```python
from build123d import *

# Parameters (mm, degrees)
SKETCH_1_W                  = 220
SKETCH_1_H                  = 220
EXTRUDE_2_DEPTH             = 220
SKETCH_3_R                  = 78
CUT_EXTRUDE_1_DEPTH         = 240
SHELL_2_T                   = 3
SKETCH_5_W                  = 207.122367347
SKETCH_5_H                  = 195.284428571
CUT_EXTRUDE_3_DEPTH         = 180
SKETCH_12_W                 = 226
SKETCH_12_H                 = 223
CUT_EXTRUDE_6_DEPTH         = 3
SKETCH_13_W                 = 226
SKETCH_13_H                 = 223
CUT_EXTRUDE_7_DEPTH         = 3
EXTRUDE_6_REACH             = 272.682
SKETCH_16_W                 = 40
SKETCH_16_H                 = 5
EXTRUDE_6_DIRECTION_2_REACH = 272.682


with BuildPart() as part:
    # 草图1 → 凸台-拉伸2 (new body)
    with BuildSketch(Plane(origin=(0, 0, 0), x_dir=(1, 0, 0), z_dir=(0, 1, 0))):
        Rectangle(SKETCH_1_W, SKETCH_1_H)
    extrude(amount=EXTRUDE_2_DEPTH)

    # 草图3 → 切除-拉伸1 (cut)
    with BuildSketch(Plane(origin=(0, 0, 0), x_dir=(1, 0, 0), z_dir=(0, 1, 0))):
        with Locations(Location((0, 0, 0), (0, 0, 270))):
            Circle(SKETCH_3_R)
    extrude(amount=CUT_EXTRUDE_1_DEPTH, mode=Mode.SUBTRACT)

    # 抽壳2
    shell_2_openings = [part.faces().sort_by_distance(p)[0] for p in [
        (0, 220, -106.888730163),
    ]]
    offset(amount=SHELL_2_T, openings=shell_2_openings, kind=Kind.INTERSECTION)

    # 草图5 → 切除-拉伸3 (cut)
    with BuildSketch(Plane.ZY.offset(-78)):
        with Locations((-1.991561224, 122.357785714)):
            Rectangle(SKETCH_5_W, SKETCH_5_H)
    extrude(amount=CUT_EXTRUDE_3_DEPTH, mode=Mode.SUBTRACT)

    # 草图12 → 切除-拉伸6 (cut)
    with BuildSketch(Plane(origin=(113, 0, 0), x_dir=(0, 0, -1), z_dir=(1, 0, 0))):
        with Locations((0, 108.5)):
            Rectangle(SKETCH_12_W, SKETCH_12_H)
    extrude(amount=-CUT_EXTRUDE_6_DEPTH, mode=Mode.SUBTRACT)

    # 草图13 → 切除-拉伸7 (cut)
    with BuildSketch(Plane.ZY.offset(113)):
        with Locations((0, 108.5)):
            Rectangle(SKETCH_13_W, SKETCH_13_H)
    extrude(amount=-CUT_EXTRUDE_7_DEPTH, mode=Mode.SUBTRACT)

    # 凸台-拉伸6: up to this face of the body (flat: up to its plane)
    extrude_6_end = Plane(part.part.faces().sort_by_distance((0, 110, -110))[0])
    # 草图16 → 凸台-拉伸6 (add, up to the picked face)
    with BuildSketch(Plane.XY, mode=Mode.PRIVATE) as extrude_6_sk1:
        with Locations((-35, 164.5)):
            Rectangle(SKETCH_16_W, SKETCH_16_H)
    extrude_6_tool1 = split(extrude(extrude_6_sk1.sketch, amount=-EXTRUDE_6_REACH, mode=Mode.PRIVATE), bisect_by=extrude_6_end, keep=Keep.BOTH, mode=Mode.PRIVATE)
    # 草图16 → 凸台-拉伸6 (add, up to the picked face)
    with BuildSketch(Plane.XY, mode=Mode.PRIVATE) as extrude_6_sk2:
        with Locations((35, 164.5)):
            Rectangle(SKETCH_16_W, SKETCH_16_H)
    extrude_6_tool2 = split(extrude(extrude_6_sk2.sketch, amount=-EXTRUDE_6_REACH, mode=Mode.PRIVATE), bisect_by=extrude_6_end, keep=Keep.BOTH, mode=Mode.PRIVATE)
    add(extrude_6_tool1.solids().sort_by(Axis((-35, 164.5, 0), (0, 0, -1)))[0])
    add(extrude_6_tool2.solids().sort_by(Axis((35, 164.5, 0), (0, 0, -1)))[0])

    # 凸台-拉伸6 direction 2: up to this face of the body (flat: up to its plane)
    extrude_6_direction_2_end = Plane(part.part.faces().sort_by_distance((0, 110, 110))[0])
    # 草图16 → 凸台-拉伸6 direction 2 (add, up to the picked face)
    with BuildSketch(Plane.XY, mode=Mode.PRIVATE) as extrude_6_direction_2_sk1:
        with Locations((-35, 164.5)):
            Rectangle(SKETCH_16_W, SKETCH_16_H)
    extrude_6_direction_2_tool1 = split(extrude(extrude_6_direction_2_sk1.sketch, amount=EXTRUDE_6_DIRECTION_2_REACH, mode=Mode.PRIVATE), bisect_by=extrude_6_direction_2_end, keep=Keep.BOTH, mode=Mode.PRIVATE)
    # 草图16 → 凸台-拉伸6 direction 2 (add, up to the picked face)
    with BuildSketch(Plane.XY, mode=Mode.PRIVATE) as extrude_6_direction_2_sk2:
        with Locations((35, 164.5)):
            Rectangle(SKETCH_16_W, SKETCH_16_H)
    extrude_6_direction_2_tool2 = split(extrude(extrude_6_direction_2_sk2.sketch, amount=EXTRUDE_6_DIRECTION_2_REACH, mode=Mode.PRIVATE), bisect_by=extrude_6_direction_2_end, keep=Keep.BOTH, mode=Mode.PRIVATE)
    add(extrude_6_direction_2_tool1.solids().sort_by(Axis((-35, 164.5, 0), (0, 0, 1)))[0])
    add(extrude_6_direction_2_tool2.solids().sort_by(Axis((35, 164.5, 0), (0, 0, 1)))[0])


solid = part.part
```
The model under review builds one solid part; all positions refer to its coordinate system, in mm. A direction names the side the tool comes from. Coordinates: 2 decimals unless noted, no trailing zeros. Write each loop counter-clockwise with the first axis right and the second up, starting at its lowest first coordinate (ties: lowest second). Pieces come first, ordered by that corner, then holes.
1) We need section B-B on x = 0. State the section outline as (y, z) points.
2) The part is to be moulded in two halves that separate along Y. For faces 1 (the face through (-2, -3, -77)), 2 (the face through (-45.636, 10.664, -59.517)), 3 (the face through (77.336, 12.185, -10.154)), say which applies: pulls with the +Y half, pulls with the -Y half, needs draft (parallel to the pull), parting line crosses it, or undercut.
3) We need section C-C on y = 197.5. State the section outline as (x, z) points.
4) We need section A-A on z = 0. State the section outline as (x, y) points, then the cut area to 3 significant figures.
5) We need section D-D on x = 33. State the section outline as (y, z) points.
6) Clearance check with flat-ended pins moving along their axes: pin 1 Ø4 at (x, z) = (9, -87) entering from +Y; pin 2 Ø4 at (y, z) = (163.5, -3) entering from -X; pin 3 Ø20 at (x, z) = (-34, 30.5) entering from +Y. State where each tip first meets the part, or that it passes through.
7) To check wall thickness, follow probe 1 along Z at (x, y) = (0, 12); probe 2 along Z at (x, y) = (50.5, 57); probe 3 along X at (y, z) = (6.25, 0). State the ranges of each line that lie inside material, in increasing order.
8) Machinability: for faces 4 (the face through (35, 167, -2)), 5 (the face through (35, 162, -2)), 6 (the face through (-2, 107, 113)), 7 (the face through (-75, 0, -26)), which of the approach directions +Z, -Z, +X, -X, +Y, -Y give a long, thin tool a straight path to every point of the face, cutting with its end or side? Answer none if there is none.
Answer list:
1. outline: (-3, -113) - (220, -113) - (220, -110) - (0, -110) - (0, -78) - (24.72, -78) - (24.72, -75) - (-3, -75) - close; (-3, 75) - (24.72, 75) - (24.72, 78) - (0, 78) - (0, 110) - (220, 110) - (220, 113) - (-3, 113) - close
2. face 1: pulls with the -Y half
2. face 2: needs draft
2. face 3: undercut
3. outline: (-110, -113) - (110, -113) - (110, -110) - (-110, -110) - close; (-110, 110) - (110, 110) - (110, 113) - (-110, 113) - close
4. outline: (-110, -3) - (-75, -3) - (-75, 24.72) - (-78, 24.72) - (-78, 0) - (-110, 0) - close; (-55, 162) - (-15, 162) - (-15, 167) - (-55, 167) - close; (15, 162) - (55, 162) - (55, 167) - (15, 167) - close; (75, -3) - (110, -3) - (110, 0) - (78, 0) - (78, 24.72) - (75, 24.72) - close
4. area: 758 mm2
5. outline: (-3, -113) - (220, -113) - (220, -110) - (167, -110) - (167, 110) - (220, 110) - (220, 113) - (-3, 113) - (-3, 67.35) - (24.72, 67.35) - (24.72, 70.68) - (0, 70.68) - (0, 110) - (162, 110) - (162, -110) - (0, -110) - (0, -70.68) - (24.72, -70.68) - (24.72, -67.35) - (-3, -67.35) - close
6. pin 1: stops at y = 0
6. pin 2: stops at x = -55
6. pin 3: stops at y = 167
7. probe 1: z = -113 to -110, -78 to -75, 75 to 78, 110 to 113
7. probe 2: z = -113 to -110, 110 to 113
7. probe 3: x = -78 to -75, 75 to 78
8. face 4: +X, -X, +Y
8. face 5: +X, -X
8. face 6: +Z, +X, -X, +Y, -Y
8. face 7: none
